Study the drawing (mm; zero at the part's minimum x, y, z) and answer. A direction names the side the tool comes from. Coordinates: 2 decimals unless noted, no trailing zeros. Loops run counter-clockwise (first coordinate to the right, second up) from the corner with the lowest first, then second, coordinate; pieces in that order, holes last.
Q1. Section A-A (x = 33.6) is taken. Give the vertices of the cut face in (y, z), then the cut area to 3 significant figures.
Q2. Section C-C (x = 58) is taken. Give the vertices of the cut face in (y, z), then the cut area to 3 significant figures.
Q3. Which of the six approach directions +Z, -Z, +X, -X, +Y, -Y give full straight-line access (tool end or side, diameter ignored) to the marked faces 4, 5 and 6?
Q4. Section D-D (z = 61) is taken. Give the vertices of the cut face in (x, y), then the cut area to 3 significant figures.
Q5. Section B-B (y = 2.25) is taken. Count the separate pieces of the cut face and the enclosed holes in it, then the cut area to 3 significant figures.
Q6. The mould has two halves that part along Z. Classify the marked faces 1, 2 and 3: pulls with the +Z half, pulls with the -Z half, needs draft (parallel to the pull), parting line crosses it, or undercut.
Q7. Straight lines are drawn through the part: line 1 (Z direction, x = 33.6, y = 1.5); line 2 (Z direction, x = 80, y = 6.5); line 3 (X direction, y = 15.5, z = 10.5). For each, find the intervals that lie inside material, in ascending order.
Q8. Flat-ended cylindrical pins translate along their axes: P1, Ø10, axis at x = 67.5, y = 10.5, coming from the -Z side; P2, Ø2.5, axis at x = 16.6, z = 13, coming from the -Y side; P3, Ø10, axis at y = 15.5, z = 17, coming from the -X side; P4, Ø4, axis at y = 2, z = 44.5, coming from the +X side. Find the tip coordinate at first contact, or state that the pin passes through.
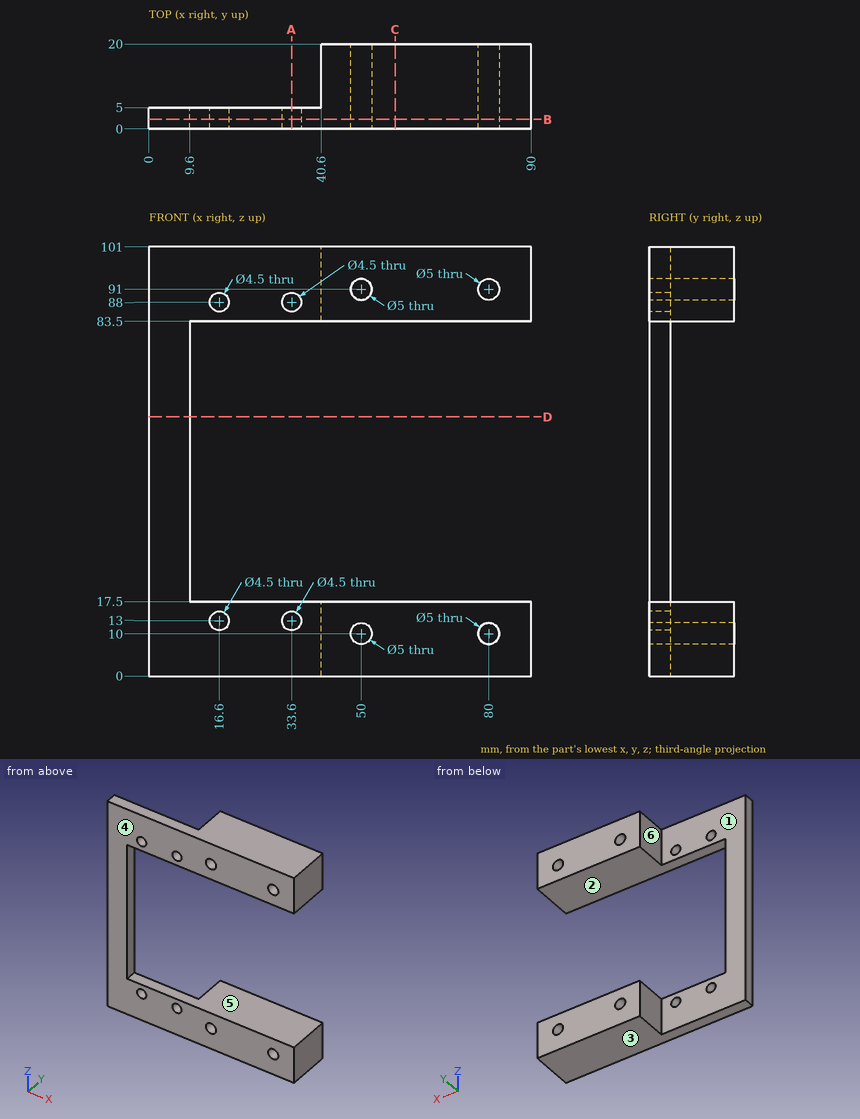
Numbers:
1. outline: (0, 0) - (5, 0) - (5, 10.75) - (0, 10.75) - close; (0, 15.25) - (5, 15.25) - (5, 17.5) - (0, 17.5) - close; (0, 83.5) - (5, 83.5) - (5, 85.75) - (0, 85.75) - close; (0, 90.25) - (5, 90.25) - (5, 101) - (0, 101) - close
1. area: 130 mm2
2. outline: (0, 0) - (20, 0) - (20, 17.5) - (0, 17.5) - close; (0, 83.5) - (20, 83.5) - (20, 101) - (0, 101) - close
2. area: 700 mm2
3. face 4: +Z, -Z, +X, -X, -Y
3. face 5: +X, +Y, -Y
3. face 6: +Z, -Z, -X, +Y
4. outline: (0, 0) - (9.6, 0) - (9.6, 5) - (0, 5) - close
4. area: 48.0 mm2
5. separate pieces: 1
5. enclosed holes: 8
5. area: 3,640 mm2
6. face 1: needs draft
6. face 2: undercut
6. face 3: pulls with the -Z half
7. line 1: z = 0 to 10.75, 15.25 to 17.5, 83.5 to 85.75, 90.25 to 101
7. line 2: z = 0 to 7.5, 12.5 to 17.5, 83.5 to 88.5, 93.5 to 101
7. line 3: x = 40.6 to 47.55, 52.45 to 77.55, 82.45 to 90
8. P1: stops at z = 0
8. P2: passes through
8. P3: stops at x = 40.6
8. P4: stops at x = 9.6
